```python
from build123d import *

# Parameters (mm, degrees)
SKETCH1_R           = 3.175
BOSS_EXTRUDE1_DEPTH = 12.7
CUT_EXTRUDE1_START  = -3.96875
SKETCH2_R           = 1.7272
CUT_EXTRUDE1_DEPTH  = 18.439134182


with BuildPart() as part:
    # Sketch1 → Boss-Extrude1 (new body)
    with BuildSketch(Plane(origin=(0, 0, 0), x_dir=(1, 0, 0), z_dir=(0, 1, 0))):
        with Locations(Location((0, 0, 0), (0, 0, 270))):
            Circle(SKETCH1_R)
    extrude(amount=BOSS_EXTRUDE1_DEPTH)

    # Sketch2 → Cut-Extrude1 (cut)
    with BuildSketch(Plane(origin=(0, 12.7, 0), x_dir=(1, 0, 0), z_dir=(0, 1, 0)).offset(CUT_EXTRUDE1_START)):
        with Locations(Location((0, 0, 0), (0, 0, 270))):
            Circle(SKETCH2_R)
    cut_extrude1 = extrude(amount=CUT_EXTRUDE1_DEPTH, mode=Mode.SUBTRACT)

    # Mirror1: Cut-Extrude1 across plane
    add(cut_extrude1.mirror(Plane.ZX.offset(6.35)), mode=Mode.SUBTRACT)


solid = part.part
```
Model file for the job. Use its own axes, mm. A direction names the side the tool comes from. Round coordinates to 2 decimals unless told otherwise and drop trailing zeros. Write each loop counter-clockwise with the first axis right and the second up, starting at its lowest first coordinate (ties: lowest second). Pieces come first, ordered by that corner, then holes. Notation, with made-up numbers: (73, -0.5) - (112, -0.5) arc R16 ccw to (112, 4.5) - close; hole circle Ø8 at (2.25, 80). An arc over 180 degrees is marked (long way). Use CSV: the item, a comma, the result in double quotes. Start each with the question number.
Item 1: Band-saw the part on D-D (y = 5.75). Write the cut outline in (x, z) (3 decimals), and give its area (3 significant figures).
Item 2: Band-saw the part on B-B (y = 10.5). Write the cut outline in (x, z) (3 decimals).
Item 3: Drill centre lines: L1, parallel to X at y = 11.5, z = 0 (3 decimals); L2, parallel to Z at x = 1.5, y = 3.75; L3, parallel to Z at x = 0.5, y = 9.75. Where is each one in solid material? Low to high. Write a range as [from, to].
Item 4: Tool access for faces 1 (the face through (-1.686, 10.688, -0.374)), 2 (the face through (0, 3.969, 0)), 3 (the face through (-1.4, 0, 1.4)): list every direction of +Z, -Z, +X, -X, +Y, -Y with a clear straight run to the whole face (end or side of a thin tool).
Item 5: Band-saw the part on A-A (z = 0). Write the cut outline in (x, y) (3 decimals).
Item 6: Band-saw the part on C-C (x = 0). Write the cut outline in (y, z) (3 decimals).
Item 7: Pin check, flat tips, straight feed: P1, Ø1, axis at y = 11, z = -1.5, coming from the -X side; P2, Ø3, axis at x = 0, z = 0, coming from the -Y side; P3, Ø1, axis at x = -2.5, y = 2.5, coming from the +Z side. Stop position of each tip, or through.
Item 8: Two-plate mould, pull along X, no slides. Class faces 4 (the face through (-1.93, 6.26, -2.52)), 5 (the face through (-1.686, 2.012, -0.374)), 6 (the face through (-1.4, 12.7, 1.4)): released by +X, released by -X, zero draft, split by the parting line, or undercut.
Checked values:
1,outline,"circle Ø6.35 at (0, 0)"
1,area,"31.7 mm²"
2,outline,"circle Ø6.35 at (0, 0); hole circle Ø3.454 at (0, 0)"
3,L1,"x = [-3.175, -1.727], [1.727, 3.175]"
3,L2,"z = [-2.8, -0.86], [0.86, 2.8]"
3,L3,"z = [-3.14, -1.65], [1.65, 3.14]"
4,face 1,"+Y"
4,face 2,"-Y"
4,face 3,"+Z, -Z, +X, -X, -Y"
5,outline,"(-3.175, 0) - (-1.727, 0) - (-1.727, 3.969) - (1.727, 3.969) - (1.727, 0) - (3.175, 0) - (3.175, 12.7) - (1.727, 12.7) - (1.727, 8.731) - (-1.727, 8.731) - (-1.727, 12.7) - (-3.175, 12.7) - close"
6,outline,"(0, -3.175) - (12.7, -3.175) - (12.7, -1.727) - (8.731, -1.727) - (8.731, 1.727) - (12.7, 1.727) - (12.7, 3.175) - (0, 3.175) - (0, 1.727) - (3.969, 1.727) - (3.969, -1.727) - (0, -1.727) - close"
7,P1,"stops at x = -3.01"
7,P2,"stops at y = 3.97"
7,P3,"stops at z = 2.47"
8,face 4,"split by the parting line"
8,face 5,"undercut"
8,face 6,"zero draft"
